from build123d import *

# Parameters (mm, degrees)
BOSS_EXTRUDE1_DEPTH = 40
CUT_EXTRUDE1_REACH  = 53.556
SKETCH2_R           = 2.5
CUT_EXTRUDE2_REACH  = 53.556
SKETCH3_R           = 2.5
FILLET1_R           = 5
SKETCH4_W           = 65
SKETCH4_H           = 80
BOSS_EXTRUDE2_DEPTH = 3
CUT_EXTRUDE3_DEPTH  = 0.5
CUT_EXTRUDE4_REACH  = 110.963
SKETCH6_R           = 1.5
CUT_EXTRUDE5_REACH  = 110.963
SKETCH7_W           = 40
SKETCH7_H           = 20


with BuildPart() as part:
    # Sketch1 → Boss-Extrude1 (new body)
    with BuildSketch(Plane.XY):
        Polygon((0, 0), (0, 23), (23, 23), (23, 20), (3, 20), (3, 0), align=None)
    extrude(amount=BOSS_EXTRUDE1_DEPTH)

    # Sketch2 → Cut-Extrude1 (cut, up to next)
    with BuildSketch(Plane(origin=(0, 23, 0), x_dir=(1, 0, 0), z_dir=(0, 1, 0)), mode=Mode.PRIVATE) as cut_extrude1_sk1:
        with Locations(Location((13, -10, 0), (0, 0, 270))):
            Circle(SKETCH2_R)
    cut_extrude1_tool1 = extrude(cut_extrude1_sk1.sketch, amount=-CUT_EXTRUDE1_REACH, mode=Mode.PRIVATE) & part.part
    # Sketch2 → Cut-Extrude1 (cut, up to next)
    with BuildSketch(Plane(origin=(0, 23, 0), x_dir=(1, 0, 0), z_dir=(0, 1, 0)), mode=Mode.PRIVATE) as cut_extrude1_sk2:
        with Locations(Location((13, -30, 0), (0, 0, 270))):
            Circle(SKETCH2_R)
    cut_extrude1_tool2 = extrude(cut_extrude1_sk2.sketch, amount=-CUT_EXTRUDE1_REACH, mode=Mode.PRIVATE) & part.part
    add(cut_extrude1_tool1.solids().sort_by_distance((13, 23, 10))[0], mode=Mode.SUBTRACT)
    add(cut_extrude1_tool2.solids().sort_by_distance((13, 23, 30))[0], mode=Mode.SUBTRACT)

    # Sketch3 → Cut-Extrude2 (cut, up to next)
    with BuildSketch(Plane.ZY, mode=Mode.PRIVATE) as cut_extrude2_sk1:
        with Locations((10, 10)):
            Circle(SKETCH3_R)
    cut_extrude2_tool1 = extrude(cut_extrude2_sk1.sketch, amount=-CUT_EXTRUDE2_REACH, mode=Mode.PRIVATE) & part.part
    # Sketch3 → Cut-Extrude2 (cut, up to next)
    with BuildSketch(Plane.ZY, mode=Mode.PRIVATE) as cut_extrude2_sk2:
        with Locations((30, 10)):
            Circle(SKETCH3_R)
    cut_extrude2_tool2 = extrude(cut_extrude2_sk2.sketch, amount=-CUT_EXTRUDE2_REACH, mode=Mode.PRIVATE) & part.part
    add(cut_extrude2_tool1.solids().sort_by_distance((0, 10, 10))[0], mode=Mode.SUBTRACT)
    add(cut_extrude2_tool2.solids().sort_by_distance((0, 10, 30))[0], mode=Mode.SUBTRACT)

    # Fillet1
    fillet1_edges = [part.edges().sort_by_distance(p)[0] for p in [
        (1.5, 0, 40),
        (1.5, 0, 0),
    ]]
    fillet(fillet1_edges, radius=FILLET1_R)

    # Sketch4 → Boss-Extrude2 (add)
    with BuildSketch(Plane(origin=(0, 23, 0), x_dir=(1, 0, 0), z_dir=(0, 1, 0))):
        with Locations((55.5, -20)):
            Rectangle(SKETCH4_W, SKETCH4_H)
    extrude(amount=-BOSS_EXTRUDE2_DEPTH)

    # Sketch5 → Cut-Extrude3 (cut)
    with BuildSketch(Plane(origin=(0, 23, 0), x_dir=(1, 0, 0), z_dir=(0, 1, 0))):
        Polygon((28.85, 14.27), (28.85, -51.73), (34.11, -51.73), (36.65, -54.27), (69.45, -54.27), (71.99, -51.73), (82.15, -51.73), (82.15, 14.27), (84.15, 16.27), (84.15, -53.73), (72.818427125, -53.73), (70.278427125, -56.27), (35.821572875, -56.27), (33.281572875, -53.73), (26.85, -53.73), (26.85, 16.27), align=None)
    extrude(amount=-CUT_EXTRUDE3_DEPTH, mode=Mode.SUBTRACT)

    # Sketch6 → Cut-Extrude4 (cut, up to next)
    with BuildSketch(Plane(origin=(0, 23, 0), x_dir=(1, 0, 0), z_dir=(0, 1, 0)), mode=Mode.PRIVATE) as cut_extrude4_sk1:
        with Locations(Location((32.15, 0.17, 0), (0, 0, 270))):
            Circle(SKETCH6_R)
    cut_extrude4_tool1 = extrude(cut_extrude4_sk1.sketch, amount=-CUT_EXTRUDE4_REACH, mode=Mode.PRIVATE) & part.part
    # Sketch6 → Cut-Extrude4 (cut, up to next)
    with BuildSketch(Plane(origin=(0, 23, 0), x_dir=(1, 0, 0), z_dir=(0, 1, 0)), mode=Mode.PRIVATE) as cut_extrude4_sk2:
        with Locations(Location((79.95, -0.93, 0), (0, 0, 270))):
            Circle(SKETCH6_R)
    cut_extrude4_tool2 = extrude(cut_extrude4_sk2.sketch, amount=-CUT_EXTRUDE4_REACH, mode=Mode.PRIVATE) & part.part
    # Sketch6 → Cut-Extrude4 (cut, up to next)
    with BuildSketch(Plane(origin=(0, 23, 0), x_dir=(1, 0, 0), z_dir=(0, 1, 0)), mode=Mode.PRIVATE) as cut_extrude4_sk3:
        with Locations(Location((64.75, -51.73, 0), (0, 0, 270))):
            Circle(SKETCH6_R)
    cut_extrude4_tool3 = extrude(cut_extrude4_sk3.sketch, amount=-CUT_EXTRUDE4_REACH, mode=Mode.PRIVATE) & part.part
    # Sketch6 → Cut-Extrude4 (cut, up to next)
    with BuildSketch(Plane(origin=(0, 23, 0), x_dir=(1, 0, 0), z_dir=(0, 1, 0)), mode=Mode.PRIVATE) as cut_extrude4_sk4:
        with Locations(Location((36.85, -51.73, 0), (0, 0, 270))):
            Circle(SKETCH6_R)
    cut_extrude4_tool4 = extrude(cut_extrude4_sk4.sketch, amount=-CUT_EXTRUDE4_REACH, mode=Mode.PRIVATE) & part.part
    add(cut_extrude4_tool1.solids().sort_by_distance((32.15, 23, -0.17))[0], mode=Mode.SUBTRACT)
    add(cut_extrude4_tool2.solids().sort_by_distance((79.95, 23, 0.93))[0], mode=Mode.SUBTRACT)
    add(cut_extrude4_tool3.solids().sort_by_distance((64.75, 23, 51.73))[0], mode=Mode.SUBTRACT)
    add(cut_extrude4_tool4.solids().sort_by_distance((36.85, 23, 51.73))[0], mode=Mode.SUBTRACT)

    # Sketch7 → Cut-Extrude5 (cut, up to next)
    with BuildSketch(Plane.ZY, mode=Mode.PRIVATE) as cut_extrude5_sk1:
        with Locations((20, 10)):
            Rectangle(SKETCH7_W, SKETCH7_H)
    cut_extrude5_tool1 = extrude(cut_extrude5_sk1.sketch, amount=-CUT_EXTRUDE5_REACH, mode=Mode.PRIVATE) & part.part
    add(cut_extrude5_tool1.solids().sort_by_distance((0, 10, 20))[0], mode=Mode.SUBTRACT)


solid = part.part
Geometry check sheet. Reference: the model listing, model coordinates, mm. A direction names the side the tool comes from. Round coordinates to 2 decimals unless told otherwise and drop trailing zeros. Loops run counter-clockwise (first coordinate to the right, second up) from the corner with the lowest first, then second, coordinate; pieces in that order, holes last. Notation, with made-up numbers: (-14, 59.25) - (11, 59.25) arc R10 ccw to (11, 74.25) - close; hole circle Ø2 at (80, 44). An arc over 180 degrees is marked (long way). Answer as CSV lines item,"result".
(1) Cross-section at B-B, the plane x = 32.15. Enter the section's corners in (y, z).
Output values:
outline,"(20, -20) - (23, -20) - (23, -1.67) - (20, -1.67) - close; (20, 1.33) - (23, 1.33) - (23, 51.73) - (22.5, 51.73) - (22.5, 53.73) - (23, 53.73) - (23, 60) - (20, 60) - close"
(2) Cross-section at C-C, the plane z = 30. Enter the section's corners in (x, y).
Output values:
outline,"(0, 20) - (10.5, 20) - (10.5, 23) - (0, 23) - close; (15.5, 20) - (88, 20) - (88, 23) - (84.15, 23) - (84.15, 22.5) - (82.15, 22.5) - (82.15, 23) - (28.85, 23) - (28.85, 22.5) - (26.85, 22.5) - (26.85, 23) - (15.5, 23) - close"
(3) Cross-section at D-D, the plane x = 13. Enter the section's corners in (y, z).
Output values:
outline,"(20, 0) - (23, 0) - (23, 7.5) - (20, 7.5) - close; (20, 12.5) - (23, 12.5) - (23, 27.5) - (20, 27.5) - close; (20, 32.5) - (23, 32.5) - (23, 40) - (20, 40) - close"
(4) Cross-section at A-A, the plane y = 21.8. Enter the section's corners in (x, z), and give its area (3 significant figures).
Output values:
outline,"(0, 0) - (23, 0) - (23, -20) - (88, -20) - (88, 60) - (23, 60) - (23, 40) - (0, 40) - close; hole circle Ø5 at (13, 10); hole circle Ø5 at (13, 30); hole circle Ø3 at (32.15, -0.17); hole circle Ø3 at (36.85, 51.73); hole circle Ø3 at (64.75, 51.73); hole circle Ø3 at (79.95, 0.93)"
area,"6,050 mm²"
(5) Set-up check for faces 1 (the face through (88, 22, 21)), 2 (the face through (23, 22, 50)), 3 (the face through (70.7, 22.75, 53.02)): record each of +Z, -Z, +X, -X, +Y, -Y from which the full face is reachable in a straight line by a thin tool's end or side.
Output values:
face 1,"+Z, -Z, +X, +Y, -Y"
face 2,"+Z, -X, +Y, -Y"
face 3,"+Y"
(6) Depth check by flat-ended pin: pin 1 Ø4 at (x, z) = (64.75, 51.73) entering from -Y; pin 2 Ø0.9 at (x, y) = (13.5, 22) entering from +Z. Enter the tip coordinate at first touch or a pass-through.
Output values:
pin 1,"stops at y = 20"
pin 2,"stops at z = 40"
(7) Material ranges on line 1 along X through (y, z) = (22.05, 51.73); line 2 along X through (y, z) = (21.9, 10); line 3 along X through (y, z) = (22.05, 0.93), recorded low to high.
Output values:
line 1,"x = 23 to 35.35, 38.35 to 63.25, 66.25 to 88"
line 2,"x = 0 to 10.5, 15.5 to 88"
line 3,"x = 0 to 31.13, 33.17 to 78.45, 81.45 to 88"
(8) Release check for a two-part mould opening along Z. For faces 4 (the face through (23, 22, -10)), 5 (the face through (66.237, 21.521, 51.535)), 6 (the face through (12, 22, 0)) record: released by +Z, released by -Z, zero draft, split by the parting line, or undercut.
Output values:
face 4,"zero draft"
face 5,"undercut"
face 6,"released by -Z"
